from build123d import *

# Parameters (mm, degrees)
F1_DEPTH = 150
F2_R     = 2.75
F3_DEPTH = 5.001


with BuildPart() as f1:
    # F0 (on Front) → F1 (new body, symmetric)
    with BuildSketch(Plane.XZ):
        with BuildLine():
            ThreePointArc((3.487119, -7.2), (6.778531, -4.248708), (8, 0))
            ThreePointArc((8, 0), (-4.248708, 6.778531), (-3.487119, -7.2))
            ThreePointArc((-3.487119, -7.2), (0, -8), (3.487119, -7.2))
        make_face()
        with BuildLine():
            ThreePointArc((3.487119, -7.2), (0, -8), (-3.487119, -7.2))
            Line((-3.487119, -7.2), (-7.008956, -13.3))
            Line((-7.008956, -13.3), (-9.25, -13.3))
            Line((-9.25, -13.3), (-9.25, -20))
            Line((-9.25, -20), (-20, -20))
            Line((-20, -20), (-20, -25))
            Line((-20, -25), (20, -25))
            Line((20, -25), (20, -20))
            Line((20, -20), (9.25, -20))
            Line((9.25, -20), (9.25, -13.3))
            Line((9.25, -13.3), (7.008956, -13.3))
            Line((7.008956, -13.3), (3.487119, -7.2))
        make_face()
    extrude(amount=F1_DEPTH, both=True)

    # F2 (on face) → F3 (cut, through all)
    with BuildSketch(Plane.XY.offset(-20)):
        with Locations((-15, -130)):
            Circle(F2_R)
        with Locations((15, -130)):
            Circle(F2_R)
        with Locations((-15, 20)):
            Circle(F2_R)
        with Locations((15, 20)):
            Circle(F2_R)
        with Locations((-15, 170)):
            Circle(F2_R)
        with Locations((15, 170)):
            Circle(F2_R)
        with Locations((-15, 320)):
            Circle(F2_R)
        with Locations((15, 320)):
            Circle(F2_R)
        with Locations((-15, 470)):
            Circle(F2_R)
        with Locations((15, 470)):
            Circle(F2_R)
        with Locations((-15, 620)):
            Circle(F2_R)
        with Locations((15, 620)):
            Circle(F2_R)
        with Locations((-15, 770)):
            Circle(F2_R)
        with Locations((15, 770)):
            Circle(F2_R)
        with Locations((-15, 920)):
            Circle(F2_R)
        with Locations((15, 920)):
            Circle(F2_R)
        with Locations((-15, 1070)):
            Circle(F2_R)
        with Locations((15, 1070)):
            Circle(F2_R)
    extrude(amount=-F3_DEPTH, mode=Mode.SUBTRACT)


solid = f1.part
Design review of the part built by this model. Coordinates are the model's own, in mm. A direction names the side the tool comes from. Give positions to 0.01 mm unless a question says otherwise; leave off trailing zeros. Order: outer loops, then holes, each group sorted by start corner. A loop starts at its lowest first (then second) coordinate and runs counter-clockwise, first axis right, second up.
1. Mouldability with a two-part tool opening along Z and no side actions: class faces 1 (the flat face through (-15, -2, -20)), 2 (the cylindrical face through (14.404, -132.685, -22.465)), 3 (the flat face through (-5.223, -2.1, -10.207)) as +Z half, -Z half, draft (parallel to the pull), parting line (faces both ways), or undercut.
Solution:
face 1: +Z half
face 2: draft
face 3: undercut
2. Add section C-C, the plane z = -16. State the section outline as (x, y) points.
Solution:
outline: (-9.25, -150) - (9.25, -150) - (9.25, 150) - (-9.25, 150) - close
3. Tool access review of faces 4 (the flat face through (5.27, -2.1, -10.29)), 5 (the flat face through (9.25, -2, -17)), 6 (the flat face through (0, 150, -12)), 7 (the cylindrical face through (-15.596, -132.685, -22.465)), 8 (the flat face through (-9.25, -2, -17)): name each direction out of +Z, -Z, +X, -X, +Y, -Y from which nothing blocks a thin tool from reaching the whole face with its end or side.
Solution:
face 4: +X, +Y, -Y
face 5: +Z, +X, +Y, -Y
face 6: +Z, -Z, +X, -X, +Y
face 7: +Z, -Z
face 8: +Z, -X, +Y, -Y
4. Add section B-B, the plane y = 121. State the section outline as (x, z) points.
Solution:
outline: (-20, -25) - (20, -25) - (20, -20) - (9.25, -20) - (9.25, -13.3) - (7.01, -13.3) - (3.49, -7.2) arc R8 ccw to (8, 0) arc R8 ccw (long way) to (-3.49, -7.2) - (-7.01, -13.3) - (-9.25, -13.3) - (-9.25, -20) - (-20, -20) - close
5. Add section A-A, the plane x = 15. State the section outline as (y, z) points.
Solution:
outline: (-150, -25) - (-132.75, -25) - (-132.75, -20) - (-150, -20) - close; (-127.25, -25) - (17.25, -25) - (17.25, -20) - (-127.25, -20) - close; (22.75, -25) - (150, -25) - (150, -20) - (22.75, -20) - close
6. To check wall thickness, follow L1, parallel to X at y = -130, z = -23.85; L2, parallel to Y at x = -15, z = -22; L3, parallel to Z at x = -17.5, y = -124.5. State the ranges of each line that lie inside material, in increasing order.
Solution:
L1: x = -20 to -17.75, -12.25 to 12.25, 17.75 to 20
L2: y = -150 to -132.75, -127.25 to 17.25, 22.75 to 150
L3: z = -25 to -20
7. For pin 1 Ø7.5 at (y, z) = (12.5, -15) entering from +X; pin 2 Ø8.5 at (x, y) = (-15.5, 53) entering from +Z; pin 3 Ø2.5 at (x, y) = (8, 38.5) entering from +Z; pin 4 Ø5 at (x, z) = (10, 3.5) entering from -Y, all flat-tipped, find the tip position at first contact; note any pin that passes through.
Solution:
pin 1: stops at x = 9.25
pin 2: stops at z = -20
pin 3: stops at z = 4.29
pin 4: passes through
